from build123d import *

# Parameters (mm, degrees)
SKETCH_1_W          = 10
SKETCH_1_H          = 10
SKETCH_1_W_2        = 7
SKETCH_1_H_2        = 7
EXTRUDE_1_DEPTH     = 85
SKETCH_2_R          = 1.6
CUT_EXTRUDE_1_DEPTH = 86.732140997
SKETCH_3_R          = 2.15
CUT_EXTRUDE_2_DEPTH = 86.732140997


with BuildPart() as part:
    # ｽｹｯﾁ1 → 押し出し-薄板1 (new body)
    with BuildSketch(Plane(origin=(0, 0, 0), x_dir=(1, 0, 0), z_dir=(0, 1, 0))):
        Rectangle(SKETCH_1_W, SKETCH_1_H)
        Rectangle(SKETCH_1_W_2, SKETCH_1_H_2, mode=Mode.SUBTRACT)
    extrude(amount=EXTRUDE_1_DEPTH)

    # ｽｹｯﾁ2 → ｶｯﾄ - 押し出し1 (cut, through all)
    with BuildSketch(Plane.XY.offset(5)):
        with Locations((0, 25)):
            Circle(SKETCH_2_R)
        with Locations((0, 5)):
            Circle(SKETCH_2_R)
        with Locations((0, 15)):
            Circle(SKETCH_2_R)
    extrude(amount=-CUT_EXTRUDE_1_DEPTH, mode=Mode.SUBTRACT)

    # ｽｹｯﾁ3 → ｶｯﾄ - 押し出し2 (cut, through all)
    with BuildSketch(Plane(origin=(5, 0, 0), x_dir=(0, 0, -1), z_dir=(1, 0, 0))):
        with Locations((0, 80)):
            Circle(SKETCH_3_R)
    extrude(amount=-CUT_EXTRUDE_2_DEPTH, mode=Mode.SUBTRACT)


solid = part.part
Could you check a few things on this model? Use its own coordinates, in mm. A direction names the side the tool comes from. Coordinates: 2 decimals unless noted, no trailing zeros. Write each loop counter-clockwise with the first axis right and the second up, starting at its lowest first coordinate (ties: lowest second). Pieces come first, ordered by that corner, then holes. Notation, with made-up numbers: M 68.25,77 L 122.25,77 A11 ccw 122.25,92 Z; hole C -15,45.5 d4. An arc over 180 degrees is marked long. One line per question, with ' | ' between items.
1) For faces 4 (the face through (0, 42, -3.5)), 5 (the face through (0, 42, -5)), which set-ups out of +Z, -Z, +X, -X, +Y, -Y let a thin tool reach every point of the face, with its end or its side?
Checks:
face 4: +Y, -Y | face 5: -Z, +X, -X, +Y, -Y
2) Imagine slicing it at C-C, the plane y = 75.5. Write out the boundary of the cut face in (x, z), and give its area (3 significant figures).
Checks:
outline: M -5,-5 L 5,-5 L 5,5 L -5,5 Z; hole M -3.5,-3.5 L 3.5,-3.5 L 3.5,3.5 L -3.5,3.5 Z | area: 51.0 mm²
3) If we mould it in two halves opening along X, with no side actions, what happens to faces 1 (the face through (4.26, 78.09, -0.99)), 2 (the face through (5, 42, 0)), 3 (the face through (3.5, 42, 0))? For each: released by +X, released by -X, zero draft, split by the parting line, or undercut.
Checks:
face 1: zero draft | face 2: released by +X | face 3: undercut
4) Imagine slicing it at A-A, the plane z = 0. Write out the boundary of the cut face in (x, y).
Checks:
outline: M -5,0 L -3.5,0 L -3.5,77.85 L -5,77.85 Z; M -5,82.15 L -3.5,82.15 L -3.5,85 L -5,85 Z; M 3.5,0 L 5,0 L 5,77.85 L 3.5,77.85 Z; M 3.5,82.15 L 5,82.15 L 5,85 L 3.5,85 Z
5) Imagine slicing it at B-B, the plane x = 0. Give the number of separate pieces and of enclosed holes in the cut face, and give its area (3 significant figures).
Checks:
separate pieces: 8 | enclosed holes: 0 | area: 226 mm²
6) Imagine slicing it at D-D, the plane y = 5. Write out the boundary of the cut face in (x, z), and give its area (3 significant figures).
Checks:
outline: M -5,-5 L -1.6,-5 L -1.6,-3.5 L -3.5,-3.5 L -3.5,3.5 L -1.6,3.5 L -1.6,5 L -5,5 Z; M 1.6,-5 L 5,-5 L 5,5 L 1.6,5 L 1.6,3.5 L 3.5,3.5 L 3.5,-3.5 L 1.6,-3.5 Z | area: 41.4 mm²
7) I need wall thicknesses on probe 1 along Y at (x, z) = (0, 4.45); probe 2 along Z at (x, y) = (-2, 68). Which ranges of each line are inside material? Lowest first, please. Write a range as [from, to].
Checks:
probe 1: [0, 3.4], [6.6, 13.4], [16.6, 23.4], [26.6, 85] | probe 2: [-5, -3.5], [3.5, 5]
8) For pin 1 Ø5 at (x, y) = (0, 25) entering from -Z; pin 2 Ø3 at (x, y) = (0, 15) entering from +Z, each with a flat end and sliding along its axis, tell me the tip position at first contact or that it passes through.
Checks:
pin 1: z = -5 | pin 2: through
